Read the model definition and answer for the solid it produces. Units are mm, in the model's axes. Give positions to 0.01 mm unless a question says otherwise; leave off trailing zeros. Order: outer loops, then holes, each group sorted by start corner. A loop starts at its lowest first (then second) coordinate and runs counter-clockwise, first axis right, second up. Notation, with made-up numbers: (-8.5, 6.25) -> (30.5, 6.25) arc R18 ccw to (30.5, 34.25) -> close; hole circle Ø8 at (43, 16). An arc over 180 degrees is marked (long way). One line per item, written item: value. Start each with the question number.
from build123d import *

# Parameters (mm, degrees)
F0_R     = 5
F1_DEPTH = 19.05
F4_R     = 25
F5_DEPTH = 25.4


# Not quite as in the source:
# - a feature of the source that left no trace in its solid (it failed there, or was rolled back) is left out


with BuildPart() as f1:
    # F0 (on Front) → F1 (new body)
    with BuildSketch(Plane.XZ):
        with BuildLine():
            ThreePointArc((0, 47.5), (-33.5875721064, -33.5875721064), (47.5, 0))
            ThreePointArc((47.5, 0), (33.5875721064, 33.5875721064), (0, 47.5))
        make_face()
        with Locations((-30.3108891325, -17.5)):
            Circle(F0_R, mode=Mode.SUBTRACT)
        with Locations((0, -35)):
            Circle(F0_R, mode=Mode.SUBTRACT)
        with Locations((30.3108891325, -17.5)):
            Circle(F0_R, mode=Mode.SUBTRACT)
        with Locations((-30.3108891325, 17.5)):
            Circle(F0_R, mode=Mode.SUBTRACT)
        with Locations((30.3108891325, 17.5)):
            Circle(F0_R, mode=Mode.SUBTRACT)
        with BuildLine():
            ThreePointArc((0, 30), (-5, 35), (0, 40))
            ThreePointArc((0, 40), (3.5355339059, 38.5355339059), (5, 35))
            ThreePointArc((5, 35), (3.5355339059, 31.4644660941), (0, 30))
        make_face(mode=Mode.SUBTRACT)
    extrude(amount=F1_DEPTH)

    # F4 (on face) → F5 (cut)
    with BuildSketch(Plane.XZ.offset(19.05)):
        Circle(F4_R)
    extrude(amount=-F5_DEPTH, mode=Mode.SUBTRACT)


solid = f1.part
Item 1: Find section C-C on z = 15. Write down the section's boundary in (x, y), then the cut area to 3 significant figures.
Item 2: Find section A-A on y = -8.5. Write down the section's boundary in (x, z), then the cut area to 3 significant figures.
Item 3: Find section D-D on z = 33. Write down the section's boundary in (x, y).
Item 4: Flat-ended cylindrical pins translate along their axes: pin 1 (9 mm diameter, centred on x = 0, z = -35, fed in from -Y); pin 2 (10 mm diameter, centred on x = 31.5, y = -11, fed in from -Z); pin 3 (1 mm diameter, centred on y = -8, z = -34.5, fed in from +X); pin 4 (3 mm diameter, centred on x = 12.5, y = -9, fed in from +Z). Find the tip coordinate at first contact, or state that the pin passes through.
Item 5: For a pull along X with two mould halves and no side action, classify faces 1 (the cylindrical face through (32.618, -9.392, 13.064)), 2 (the flat face through (20, -19.05, -20)), 3 (the cylindrical face through (32.618, -9.392, -21.936)) as +X half, -X half, draft (parallel to the pull), parting line (faces both ways), or undercut.
Item 6: Find the intervals of material crossed by line 1 (X direction, y = -16.5, z = 20); line 2 (X direction, y = -1.75, z = -19); line 3 (Z direction, x = 28.5, y = -15.75), in increasing order. Write a range as from..to.
Item 7: Find section B-B on x = 29. Write down the section's boundary in (y, z), then the cut area to 3 significant figures.
Checks:
1. outline: (-45.07, -19.05) -> (-34.64, -19.05) -> (-34.64, 0) -> (-45.07, 0) -> close; (-25.98, -19.05) -> (-20, -19.05) -> (-20, 0) -> (-25.98, 0) -> close; (20, -19.05) -> (25.98, -19.05) -> (25.98, 0) -> (20, 0) -> close; (34.64, -19.05) -> (45.07, -19.05) -> (45.07, 0) -> (34.64, 0) -> close
1. area: 625 mm2
2. outline: circle Ø95 at (0, 0); hole circle Ø10 at (-30.31, -17.5); hole circle Ø10 at (-30.31, 17.5); hole circle Ø50 at (0, 0); hole circle Ø10 at (0, -35); hole circle Ø10 at (0, 35); hole circle Ø10 at (30.31, -17.5); hole circle Ø10 at (30.31, 17.5)
2. area: 4,650 mm2
3. outline: (-34.17, -19.05) -> (-4.58, -19.05) -> (-4.58, 0) -> (-34.17, 0) -> close; (4.58, -19.05) -> (34.17, -19.05) -> (34.17, 0) -> (4.58, 0) -> close
4. pin 1: through
4. pin 2: z = -39.42
4. pin 3: x = 33.17
4. pin 4: z = 46.21
5. face 1: undercut
5. face 2: draft
5. face 3: undercut
6. line 1: -43.08..-34.64, -25.98..-15, 15..25.98, 34.64..43.08
6. line 2: -43.53..-35.08, -25.54..-16.25, 16.25..25.54, 35.08..43.53
6. line 3: -38..-22.16, -12.84..12.84, 22.16..38
7. outline: (-19.05, -37.62) -> (0, -37.62) -> (0, -22.33) -> (-19.05, -22.33) -> close; (-19.05, -12.67) -> (0, -12.67) -> (0, 12.67) -> (-19.05, 12.67) -> close; (-19.05, 22.33) -> (0, 22.33) -> (0, 37.62) -> (-19.05, 37.62) -> close
7. area: 1,070 mm2
